from build123d import *

# Parameters (mm, degrees)
F0_W      = 23
F0_H      = 49
F1_DEPTH  = 1.5
F2_W      = 23
F2_H      = 1.5
F3_DEPTH  = 22
F4_W      = 2
F4_H      = 1
F5_DEPTH  = 22
F6_W      = 47
F6_H      = 21.5
F7_DEPTH  = 1.5
F8_W      = 1.5
F8_H      = 49
F9_DEPTH  = 23.5
F11_DEPTH = 10
F12_W     = 6
F12_H     = 10
F13_DEPTH = 1.5
F14_W     = 2
F14_H     = 1.5
F15_DEPTH = 2
F16_W     = 8
F16_H     = 6.5
F17_DEPTH = 2.2
F18_W     = 45.5
F18_H     = 1.5
F19_DEPTH = 5
F20_W     = 45.5
F20_H     = 1.5
F21_DEPTH = 5
F22_R     = 5


with BuildPart() as f1:
    # F0 (on Top) → F1 (new body)
    with BuildSketch(Plane.XY):
        with Locations((-11.5, 0)):
            Rectangle(F0_W, F0_H)
    extrude(amount=F1_DEPTH)

    # F2 (on face) → F3 (join)
    with BuildSketch(Plane.XY.offset(1.5)):
        with Locations((-11.5, 23.75)):
            Rectangle(F2_W, F2_H)
        with Locations((-11.5, -23.75)):
            Rectangle(F2_W, F2_H)
    extrude(amount=F3_DEPTH)

    # F4 (on face) → F5 (join)
    with BuildSketch(Plane.XY.offset(1.5)):
        with Locations((-4, 22.5)):
            Rectangle(F4_W, F4_H)
        with Locations((-8, -22.5)):
            Rectangle(F4_W, F4_H)
        with Locations((-4, -22.5)):
            Rectangle(F4_W, F4_H)
        with Locations((-8, 22.5)):
            Rectangle(F4_W, F4_H)
    extrude(amount=F5_DEPTH)

    # F6 (on Top) → F7 (join)
    with BuildSketch(Plane.XY):
        with Locations((23.5, 0)):
            Rectangle(F6_W, F6_H)
    extrude(amount=F7_DEPTH)

    # F8 (on Top) → F9 (join)
    with BuildSketch(Plane.XY):
        with Locations((0.75, 0)):
            Rectangle(F8_W, F8_H)
    extrude(amount=F9_DEPTH)

    # F10 (on face) → F11 (join)
    with BuildSketch(Plane.XY.offset(1.5)):
        Polygon((1.5, 10.75), (1.5, 8.9), (44.8, 8.9), (44.8, -8.9), (1.5, -8.9), (1.5, -10.75), (47, -10.75), (47, 10.75), align=None)
    extrude(amount=F11_DEPTH)

    # F12 (on face) → F13 (cut, through all)
    with BuildSketch(Plane(origin=(0, 0, 0), x_dir=(0, -1, 0), z_dir=(-1, 0, 0))):
        with Locations((0, 6.5)):
            Rectangle(F12_W, F12_H)
    extrude(amount=-F13_DEPTH, mode=Mode.SUBTRACT)

    # F14 (on face) → F15 (join)
    with BuildSketch(Plane.XY.offset(1.5)):
        with Locations((2.5, 8.15)):
            Rectangle(F14_W, F14_H)
        with Locations((2.5, -8.15)):
            Rectangle(F14_W, F14_H)
        with Locations((43.8, 8.15)):
            Rectangle(F14_W, F14_H)
        with Locations((43.8, -8.15)):
            Rectangle(F14_W, F14_H)
    extrude(amount=F15_DEPTH)

    # F16 (on face) → F17 (cut, through all)
    with BuildSketch(Plane.YZ.offset(47)):
        with Locations((0, 8.25)):
            Rectangle(F16_W, F16_H)
    extrude(amount=-F17_DEPTH, mode=Mode.SUBTRACT)

    # F18 (on face) → F19 (join)
    with BuildSketch(Plane(origin=(0, 10.75, 0), x_dir=(-1, 0, 0), z_dir=(0, 1, 0))):
        with Locations((-24.25, 0.75)):
            Rectangle(F18_W, F18_H)
    extrude(amount=F19_DEPTH)

    # F20 (on face) → F21 (join)
    with BuildSketch(Plane.XZ.offset(10.75)):
        with Locations((24.25, 0.75)):
            Rectangle(F20_W, F20_H)
    extrude(amount=F21_DEPTH)

    # F22
    f22_edges = [f1.edges().sort_by_distance(p)[0] for p in [
        (47, 15.75, 0.75),
        (1.5, 15.75, 0.75),
        (47, -15.75, 0.75),
        (1.5, -15.75, 0.75),
    ]]
    fillet(f22_edges, radius=F22_R)


solid = f1.part
The listing builds one solid part. Answer for the finished solid, in the listing's coordinates (mm). A direction names the side the tool comes from. Round coordinates to 2 decimals unless told otherwise and drop trailing zeros. Order: outer loops, then holes, each group sorted by start corner. A loop starts at its lowest first (then second) coordinate and runs counter-clockwise, first axis right, second up. Notation, with made-up numbers: (-38.5, 4.25) - (-16.5, 4.25) arc R11 ccw to (-16.5, 10.25) - close; hole circle Ø3 at (59, -1.75). An arc over 180 degrees is marked (long way). Write item = value, one per line. Start each with the question number.
1) For a pull along Z with two mould halves and no side action, classify faces 5 (the flat face through (1, 3, 6)), 6 (the flat face through (24, -15.75, 1)), 7 (the flat face through (2, 8, 3.5)) as released by +Z, released by -Z, zero draft, split by the parting line, or undercut.
2) Section A-A, the plane y = 0 is taken. Write down the section's boundary in (x, z).
3) For faces 1 (the flat face through (-2, 23, 12)), 2 (the flat face through (-4, -22, 12)), 3 (the flat face through (24, -10.75, 6)), 4 (the flat face through (24, 15.75, 1)), determine the directions among +Z, -Z, +X, -X, +Y, -Y from which every point of the face is accessible in a straight line to the end or side of a thin tool.
4) Section D-D, the plane y = 6.5 is taken. Write down the section's boundary in (x, z).
5) Section B-B, the plane z = 17.25 is taken. Write down the section's boundary in (x, y), plus the area to 4 significant figures.
6) Section C-C, the plane x = 11 is taken. Write down the section's boundary in (y, z), plus the area to 4 significant figures.
7) Given pin 1 (8 mm diameter, centred on x = 17, z = 3, fed in from +Y); pin 2 (8 mm diameter, centred on x = 22.5, y = -5, fed in from +Z); pin 3 (2 mm diameter, centred on x = 21, y = -6, fed in from +Z), each flat-ended and moving along its own axis, determine where each tip first touches the part or whether it passes through.
8) Straight lines are drawn through the part: L1, parallel to Y at x = -12, z = 16.75; L2, parallel to X at y = -4, z = 21.25; L3, parallel to Y at x = 42, z = 6.5. For each, find the intervals that lie inside material, in ascending order.
Results list:
q1.face_5 = undercut
q1.face_6 = zero draft
q1.face_7 = released by +Z
q2.outline = (-23, 0) - (47, 0) - (47, 5) - (44.8, 5) - (44.8, 1.5) - (-23, 1.5) - close; (0, 11.5) - (1.5, 11.5) - (1.5, 23.5) - (0, 23.5) - close
q3.face_1 = +Z
q3.face_2 = +Z, -X
q3.face_3 = +Z, +X, -Y
q3.face_4 = +Z, -Z, +X, +Y
q4.outline = (-23, 0) - (47, 0) - (47, 11.5) - (44.8, 11.5) - (44.8, 1.5) - (1.5, 1.5) - (1.5, 23.5) - (0, 23.5) - (0, 1.5) - (-23, 1.5) - close
q5.outline = (-23, -24.5) - (1.5, -24.5) - (1.5, 24.5) - (-23, 24.5) - (-23, 23) - (-9, 23) - (-9, 22) - (-7, 22) - (-7, 23) - (-5, 23) - (-5, 22) - (-3, 22) - (-3, 23) - (0, 23) - (0, -23) - (-3, -23) - (-3, -22) - (-5, -22) - (-5, -23) - (-7, -23) - (-7, -22) - (-9, -22) - (-9, -23) - (-23, -23) - close
q5.area = 150.5 mm^2
q6.outline = (-15.75, 0) - (15.75, 0) - (15.75, 1.5) - (10.75, 1.5) - (10.75, 11.5) - (8.9, 11.5) - (8.9, 1.5) - (-8.9, 1.5) - (-8.9, 11.5) - (-10.75, 11.5) - (-10.75, 1.5) - (-15.75, 1.5) - close
q6.area = 84.25 mm^2
q7.pin_1 = 15.75
q7.pin_2 = 11.5
q7.pin_3 = 1.5
q8.L1 = -24.5 to -23, 23 to 24.5
q8.L2 = 0 to 1.5
q8.L3 = -10.75 to -8.9, 8.9 to 10.75
